Check sheet for the modelled part. Datum: model origin and axes. Units: mm. A direction names the side the tool comes from. Give positions to 0.01 mm unless a question says otherwise; leave off trailing zeros. Order: outer loops, then holes, each group sorted by start corner. A loop starts at its lowest first (then second) coordinate and runs counter-clockwise, first axis right, second up.
from build123d import *

# Parameters (mm, degrees)
SKETCH1_W                = 35
SKETCH1_H                = 20
BOSS_EXTRUDE1_DEPTH      = 3
M8_CLEARANCE_SLOT1_DEPTH = 3
M4_CLEARANCE_SLOT1_D     = 4.5


# Read off the part's stored shape, not the designer's step: M8 Clearance Slot1
with BuildPart() as part:
    # Sketch1 → Boss-Extrude1 (new body)
    with BuildSketch(Plane(origin=(0, 0, 0), x_dir=(1, 0, 0), z_dir=(0, 1, 0))):
        with Locations((-7.459731544, -5.86409396)):
            Rectangle(SKETCH1_W, SKETCH1_H)
    extrude(amount=BOSS_EXTRUDE1_DEPTH)

    # M8 Clearance Slot1 outline → M8 Clearance Slot1 (cut)
    with BuildSketch(Plane(origin=(0, 0, 0), x_dir=(1, 0, 0), z_dir=(0, 1, 0))):
        with BuildLine():
            Line((-8.959731544, -10.36409396), (3.040268456, -10.36409396))
            ThreePointArc((3.040268456, -10.36409396), (7.540268456, -5.86409396), (3.040268456, -1.36409396))
            Line((3.040268456, -1.36409396), (-8.959731544, -1.36409396))
            ThreePointArc((-8.959731544, -1.36409396), (-13.459731544, -5.86409396), (-8.959731544, -10.36409396))
        make_face()
    extrude(amount=M8_CLEARANCE_SLOT1_DEPTH, mode=Mode.SUBTRACT)

    # M4 Clearance Slot1 (through all)
    with Locations(Plane(origin=(0, 3, 0), x_dir=(1, 0, 0), z_dir=(0, 1, 0))):
        with Locations((-19.459731544, -5.86409396)):
            Hole(M4_CLEARANCE_SLOT1_D / 2)


solid = part.part
1) Draft check along X on faces 3 (the face through (-8, 1, 15.864)), 4 (the face through (-13.46, 1.48, 5.77)), 5 (the face through (-24.96, 1, 6)). Enter one of: +X half, -X half, draft (parallel to the pull), parting line (faces both ways), or undercut.
Recorded:
face 3: draft
face 4: undercut
face 5: -X half
2) Section check D-D, the plane y = 2.6. Record the cut outline in (x, z).
Recorded:
outline: (-24.96, -4.14) - (10.04, -4.14) - (10.04, 15.86) - (-24.96, 15.86) - close; hole circle Ø4.5 at (-19.46, 5.86); hole (-8.96, 1.36) - (3.04, 1.36) arc R4.5 ccw to (3.04, 10.36) - (-8.96, 10.36) arc R4.5 ccw to start
3) Section check C-C, the plane z = 6.75. Record the cut outline in (x, y).
Recorded:
outline: (-24.96, 0) - (-21.53, 0) - (-21.53, 3) - (-24.96, 3) - close; (-17.39, 0) - (-13.37, 0) - (-13.37, 3) - (-17.39, 3) - close; (7.45, 0) - (10.04, 0) - (10.04, 3) - (7.45, 3) - close
4) Material ranges on L1, parallel to X at y = 2.7, z = 6; L2, parallel to Z at x = -7, y = 1.7; L3, parallel to X at y = 0.3, z = 7, recorded low to high.
Recorded:
L1: x = -24.96 to -21.71, -17.21 to -13.46, 7.54 to 10.04
L2: z = -4.14 to 1.36, 10.36 to 15.86
L3: x = -24.96 to -21.4, -17.52 to -13.31, 7.39 to 10.04
5) Section check A-A, the plane x = -1.5. Record the cut outline in (y, z).
Recorded:
outline: (0, -4.14) - (3, -4.14) - (3, 1.36) - (0, 1.36) - close; (0, 10.36) - (3, 10.36) - (3, 15.86) - (0, 15.86) - close
6) Set-up check for faces 1 (the face through (-3, 1, 1.364)), 2 (the face through (-8, 0, 1)): record each of +Z, -Z, +X, -X, +Y, -Y from which the full face is reachable in a straight line by a thin tool's end or side.
Recorded:
face 1: +Y, -Y
face 2: +Z, -Z, +X, -X, -Y
7) Section check B-B, the plane z = 2.5. Record the cut outline in (x, y).
Recorded:
outline: (-24.96, 0) - (-11.95, 0) - (-11.95, 3) - (-24.96, 3) - close; (6.03, 0) - (10.04, 0) - (10.04, 3) - (6.03, 3) - close
